The drawing under review shows one solid part. Ordinate dimensions are in mm from its lowest x, y, z. Coordinates: 2 decimals unless noted, no trailing zeros. Loops run counter-clockwise (first coordinate to the right, second up) from the corner with the lowest first, then second, coordinate; pieces in that order, holes last.
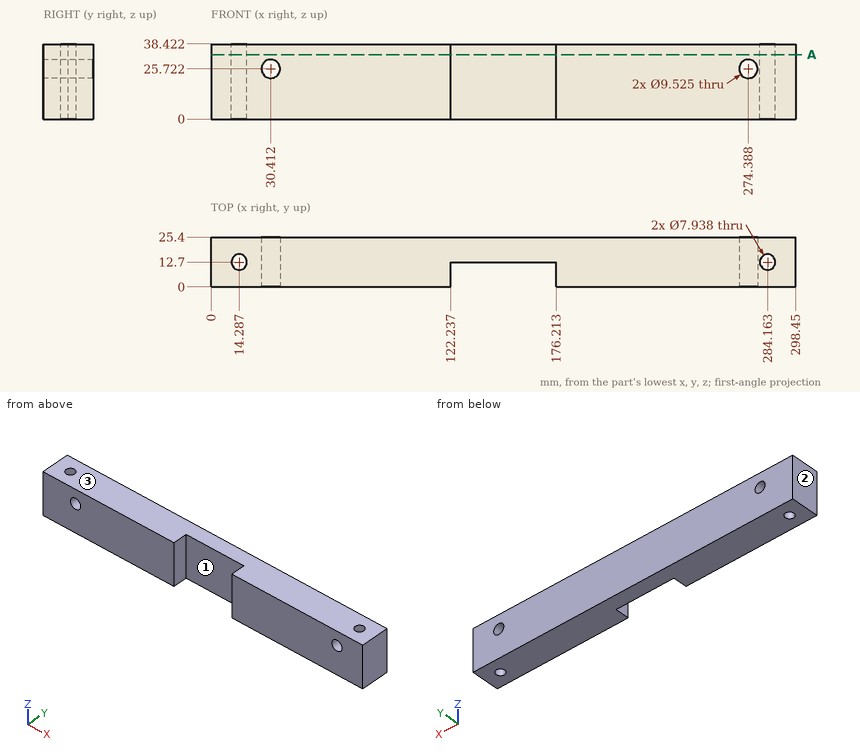
Q1. The part is to be moulded in two halves that separate along X. For the marked faces 1, 2 and 3, say which applies: pulls with the +X half, pulls with the -X half, needs draft (parallel to the pull), parting line crosses it, or undercut.
Q2. Take a section at A-A, the plane z = 33. Write out the cut boundary in (x, y), then the cut area to 3 significant figures.
Q3. For line 1 (X direction, y = 8.25, z = 32); line 2 (Y direction, x = 135.5, z = 14.5), list the stretches that pass through material, from the lowest coordinate up.
Q4. Clearance check with flat-ended pins moving along their axes: pin 1 Ø19 at (x, z) = (158, 21) entering from -Y; pin 2 Ø8.5 at (x, z) = (30.41, 25.72) entering from -Y. State where each tip first meets the part, or that it passes through.
Entries:
1. face 1: undercut
1. face 2: pulls with the -X half
1. face 3: needs draft
2. outline: (0, 0) - (122.24, 0) - (122.24, 12.7) - (176.21, 12.7) - (176.21, 0) - (298.45, 0) - (298.45, 25.4) - (0, 25.4) - close; hole circle Ø7.94 at (14.29, 12.7); hole circle Ø7.94 at (284.16, 12.7)
2. area: 6,800 mm2
3. line 1: x = 0 to 122.24, 176.21 to 298.45
3. line 2: y = 12.7 to 25.4
4. pin 1: stops at y = 12.7
4. pin 2: passes through
